The model under review builds one solid part; all positions refer to its coordinate system, in mm. Face numbers are marked on the shaded views. A direction names the side the tool comes from. Coordinates: 2 decimals unless noted, no trailing zeros. Order: outer loops, then holes, each group sorted by start corner. A loop starts at its lowest first (then second) coordinate and runs counter-clockwise, first axis right, second up. Notation, with made-up numbers: (-35, -39.75) - (19, -39.75) arc R25 ccw to (19, -6.75) - close; hole circle Ø5 at (74.25, 64). An arc over 180 degrees is marked (long way). Answer in a Markdown table with one row per item.
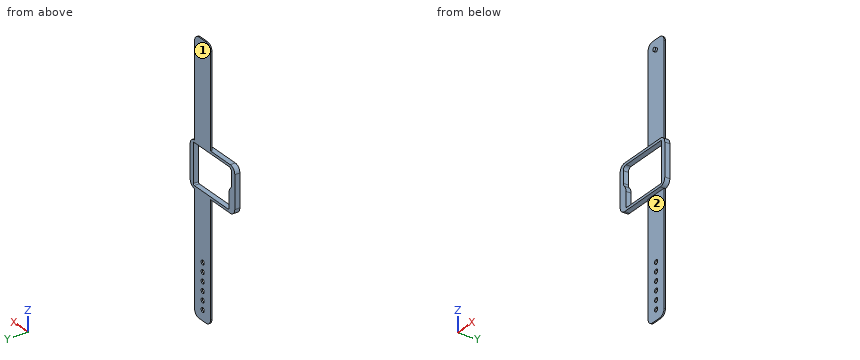
```python
from build123d import *

# Parameters (mm, degrees)
SKETCH1_R           = 1.75
BOSS_EXTRUDE1_DEPTH = 1
FILLET1_R           = 5
BOSS_EXTRUDE2_START = 3
SKETCH2_W           = 50
SKETCH2_H           = 35.75
BOSS_EXTRUDE2_DEPTH = 3
FILLET3_R           = 1
SKETCH4_R           = 1.5
BOSS_EXTRUDE3_DEPTH = 2.5
BOSS_EXTRUDE4_START = -1
SKETCH5_R           = 1.75
BOSS_EXTRUDE4_DEPTH = 1
FILLET8_R           = 5


with BuildPart() as part:
    # Sketch1 → Boss-Extrude1 (new body)
    with BuildSketch(Plane(origin=(0, 0, 0), x_dir=(1, 0, 0), z_dir=(0, 1, 0))):
        Polygon((-27, 2), (0, 2), (0, 95.3), (18, 95.3), (18, 2), (23, 2), (23, -33.75), (18, -33.75), (18, -111.75), (0, -111.75), (0, -33.75), (-27, -33.75), align=None)
        with Locations(Location((9, -103.75, 0), (0, 0, 270))):
            Circle(SKETCH1_R, mode=Mode.SUBTRACT)
        with Locations(Location((9, 87.3, 0), (0, 0, 270))):
            Circle(SKETCH1_R, mode=Mode.SUBTRACT)
        with Locations(Location((9, 80.3, 0), (0, 0, 270))):
            Circle(SKETCH1_R, mode=Mode.SUBTRACT)
        with Locations(Location((9, 73.3, 0), (0, 0, 270))):
            Circle(SKETCH1_R, mode=Mode.SUBTRACT)
        with Locations(Location((9, 66.3, 0), (0, 0, 270))):
            Circle(SKETCH1_R, mode=Mode.SUBTRACT)
        with Locations(Location((9, 59.3, 0), (0, 0, 270))):
            Circle(SKETCH1_R, mode=Mode.SUBTRACT)
        with Locations(Location((9, 52.3, 0), (0, 0, 270))):
            Circle(SKETCH1_R, mode=Mode.SUBTRACT)
        with BuildLine():
            Line((-23.5, -28.75), (-23.5, -19.49269966))
            ThreePointArc((-23.5, -19.49269966), (-23.215880477, -18.058623358), (-22.406445692, -16.841202283))
            ThreePointArc((-22.406445692, -16.841202283), (-20.995319195, -14.718813714), (-20.5, -12.218719692))
            Line((-20.5, -12.218719692), (-20.5, 0))
            Line((-20.5, 0), (19.5, 0))
            Line((19.5, 0), (19.5, -31.75))
            Line((19.5, -31.75), (-20.5, -31.75))
            ThreePointArc((-20.5, -31.75), (-22.621320344, -30.871320344), (-23.5, -28.75))
        make_face(mode=Mode.SUBTRACT)
    extrude(amount=BOSS_EXTRUDE1_DEPTH)

    # Fillet1
    fillet1_edges = [part.edges().sort_by_distance(p)[0] for p in [
        (18, 0.5, 111.75),
        (0, 0.5, 111.75),
        (0, 0.5, -95.3),
        (18, 0.5, -95.3),
    ]]
    fillet(fillet1_edges, radius=FILLET1_R)

    # Sketch2 → Boss-Extrude2 (add)
    with BuildSketch(Plane.XZ.offset(BOSS_EXTRUDE2_START)):
        with Locations((-2, 15.875)):
            Rectangle(SKETCH2_W, SKETCH2_H)
        with BuildLine():
            ThreePointArc((-22.406445692, 16.841202283), (-23.215880477, 18.058623358), (-23.5, 19.49269966))
            Line((-23.5, 19.49269966), (-23.5, 28.75))
            ThreePointArc((-23.5, 28.75), (-22.621320344, 30.871320344), (-20.5, 31.75))
            Line((-20.5, 31.75), (19.5, 31.75))
            Line((19.5, 31.75), (19.5, 0))
            Line((19.5, 0), (-20.5, 0))
            Line((-20.5, 0), (-20.5, 12.218719692))
            ThreePointArc((-20.5, 12.218719692), (-20.995319195, 14.718813714), (-22.406445692, 16.841202283))
        make_face(mode=Mode.SUBTRACT)
    extrude(amount=-BOSS_EXTRUDE2_DEPTH)

    # Fillet3
    fillet3_edges = [part.edges().sort_by_distance(p)[0] for p in [
        (-20.5, -1, 0),
        (19.5, -1, 31.75),
        (19.5, -1, 0),
    ]]
    fillet(fillet3_edges, radius=FILLET3_R)



with BuildPart() as body_2:
    # Sketch4 → Boss-Extrude3 (new body)
    with BuildSketch(Plane(origin=(0, 1, 0), x_dir=(1, 0, 0), z_dir=(0, 1, 0))):
        with Locations(Location((9, -103.75, 0), (0, 0, 270))):
            Circle(SKETCH4_R)
    extrude(amount=-BOSS_EXTRUDE3_DEPTH)


with BuildPart() as part_1:
    add(part.part)

    add(body_2.part)  # Boss-Extrude4 merges body 2
    # Sketch5 → Boss-Extrude4 (add)
    with BuildSketch(Plane(origin=(0, 1, 0), x_dir=(1, 0, 0), z_dir=(0, 1, 0)).offset(BOSS_EXTRUDE4_START)):
        with Locations((9, -103.75)):
            Circle(SKETCH5_R)
    extrude(amount=BOSS_EXTRUDE4_DEPTH)

    # Fillet8
    fillet8_edges = [part_1.edges().sort_by_distance(p)[0] for p in [
        (23, -1, -2),
        (23, -1, 33.75),
        (-27, -1, 33.75),
        (-27, -1, -2),
    ]]
    fillet(fillet8_edges, radius=FILLET8_R - 0.0001)  # a hair under: the kernel refuses the full size


solid = part_1.part
```
Item 1: We need section B-B, the plane z = 5. Write out the cut boundary in (x, y).
Check values:
| item | result |
|---|---|
| outline | (-27, -3) - (-20.5, -3) - (-20.5, 1) - (-27, 1) - close; (19.5, -3) - (23, -3) - (23, 1) - (19.5, 1) - close |
Item 2: Clearance check with flat-ended pins moving along their axes: pin 1 Ø0.8 at (y, z) = (0.5, 88) entering from +X; pin 2 Ø1.5 at (y, z) = (-0.5, 54) entering from -X; pin 3 Ø2 at (x, y) = (-5.5, -1.5) entering from +Z. State where each tip first meets the part, or that it passes through.
Check values:
| item | result |
|---|---|
| pin 1 | x = 18 |
| pin 2 | x = 0 |
| pin 3 | z = 33.75 |
Item 3: We need section D-D, the plane x = 15. Write out the cut boundary in (y, z).
Check values:
| item | result |
|---|---|
| outline | (-3, -2) - (0, -2) - (0, -94.88) - (1, -94.88) - (1, 0) - (-3, 0) - close; (-3, 31.75) - (1, 31.75) - (1, 111.33) - (0, 111.33) - (0, 33.75) - (-3, 33.75) - close |
Item 4: To check wall thickness, follow line 1 (Z direction, x = 12.5, y = -0.2); line 2 (X direction, y = 0.35, z = -87.3); line 3 (X direction, y = -1.65, z = 9.5). State the ranges of each line that lie inside material, in increasing order. Write a range as from..to.
Check values:
| item | result |
|---|---|
| line 1 | -2..0, 31.75..33.75 |
| line 2 | 0..7.25, 10.75..18 |
| line 3 | -27..-20.5, 19.5..23 |
Item 5: We need section A-A, the plane y = -0.7. Write out the cut boundary in (x, z).
Check values:
| item | result |
|---|---|
| outline | (-27, 3) arc R5 ccw to (-22, -2) - (18, -2) arc R5 ccw to (23, 3) - (23, 28.75) arc R5 ccw to (18, 33.75) - (-22, 33.75) arc R5 ccw to (-27, 28.75) - close; circle Ø3 at (9, 103.75); hole (-23.5, 19.49) arc R3.76 ccw to (-22.41, 16.84) arc R6.56 cw to (-20.5, 12.22) - (-20.5, 1) arc R1 ccw to (-19.5, 0) - (18.5, 0) arc R1 ccw to (19.5, 1) - (19.5, 30.75) arc R1 ccw to (18.5, 31.75) - (-20.5, 31.75) arc R3 ccw to (-23.5, 28.75) - close |
Item 6: Tool access review of the marked faces 1 and 2: name each direction out of +Z, -Z, +X, -X, +Y, -Y from which nothing blocks a thin tool from reaching the whole face with its end or side.
Check values:
| item | result |
|---|---|
| face 1 | +Z, -Z, +X, -X, +Y |
| face 2 | -Z, +X, -X, -Y |
Item 7: We need section C-C, the plane x = -5.5. Write out the cut boundary in (y, z), then the cut area to 3 significant figures.
Check values:
| item | result |
|---|---|
| outline | (-3, -2) - (1, -2) - (1, 0) - (-3, 0) - close; (-3, 31.75) - (1, 31.75) - (1, 33.75) - (-3, 33.75) - close |
| area | 16.0 mm^2 |
